Here's the drawing with two shaded views (mm, measured from the low corner). I have some questions. Coordinates: 2 decimals unless noted, no trailing zeros. Write each loop counter-clockwise with the first axis right and the second up, starting at its lowest first coordinate (ties: lowest second). Pieces come first, ordered by that corner, then holes. Notation, with made-up numbers: (56, 5.5) -> (108, 5.5) arc R32 cw to (108, 33.5) -> close; hole circle Ø11 at (87.5, 23.5). An arc over 180 degrees is marked (long way). Use one line per item in the form item = value.
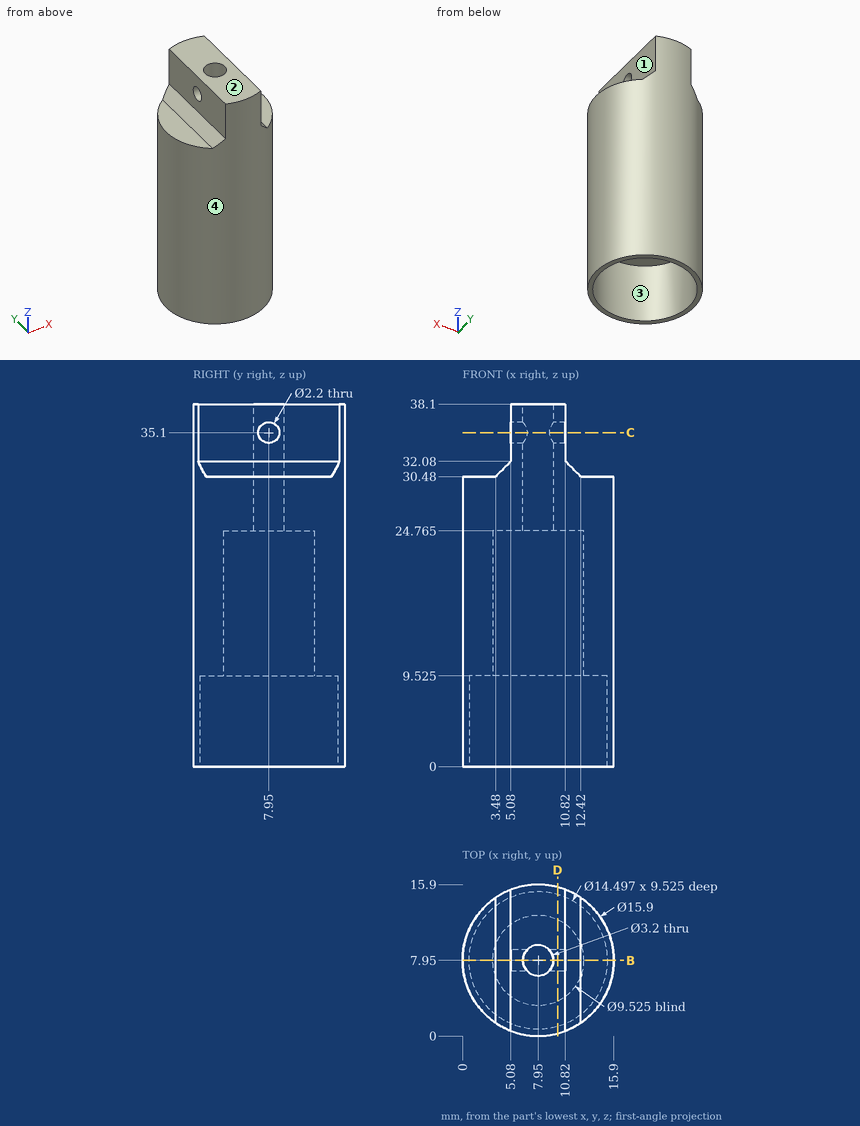
Q1. Suppose I cut it at C-C (z = 35.1). Write out the boundary of the cut face in (x, y), then the cut area to 3 significant figures.
Return value:
outline = (5.08, 0.54) arc R7.95 ccw to (10.82, 0.54) -> (10.82, 6.85) -> (9.11, 6.85) arc R1.6 cw to (6.79, 6.85) -> (5.08, 6.85) -> close; (5.08, 9.05) -> (6.79, 9.05) arc R1.6 cw to (9.11, 9.05) -> (10.82, 9.05) -> (10.82, 15.36) arc R7.95 ccw to (5.08, 15.36) -> close
area = 75.0 mm2
Q2. Suppose I cut it at B-B (y = 7.95). Give the number of separate pieces and of enclosed holes in the cut face, then the cut area to 3 significant figures.
Return value:
separate_pieces = 4
enclosed_holes = 0
area = 199 mm2
Q3. Suppose I cut it at D-D (x = 10). Write out the boundary of the cut face in (y, z) (3 decimals).
Return value:
outline = (0.269, 0) -> (0.997, 0) -> (0.997, 9.525) -> (3.651, 9.525) -> (3.651, 24.765) -> (12.249, 24.765) -> (12.249, 9.525) -> (14.903, 9.525) -> (14.903, 0) -> (15.631, 0) -> (15.631, 38.1) -> (0.269, 38.1) -> close; hole circle Ø2.2 at (7.95, 35.1)
Q4. Thinking about a two-plate mould opening in X: for the marked faces 1, 2, 3 and 4, which applies, released by +X, released by -X, zero draft, split by the parting line, or undercut?
Return value:
face_1 = released by +X
face_2 = zero draft
face_3 = undercut
face_4 = split by the parting line
Q5. If I drill on line 1 (X direction, y = 7.95, z = 33.5); line 2 (X direction, y = 7.95, z = 28); line 3 (Z direction, x = 5.7, y = 7.95) (3 decimals), over which ranges is the centre line in solid material (lowest first)? Write a range as from..to.
Return value:
line_1 = 5.08..6.35, 9.55..10.82
line_2 = 0..6.35, 9.55..15.9
line_3 = 24.765..34, 36.2..38.1
Q6. Will these pins go through, and if not, where does the flat tip stop? pin 1 (2 mm diameter, centred on x = 7, y = 4, fed in from -Z) (3 decimals); pin 2 (3 mm diameter, centred on x = 9, y = 5.5, fed in from -Z) (3 decimals); pin 3 (5 mm diameter, centred on y = 9.5, z = 36.5, fed in from -X).
Return value:
pin_1 = 9.525
pin_2 = 24.765
pin_3 = 5.08
